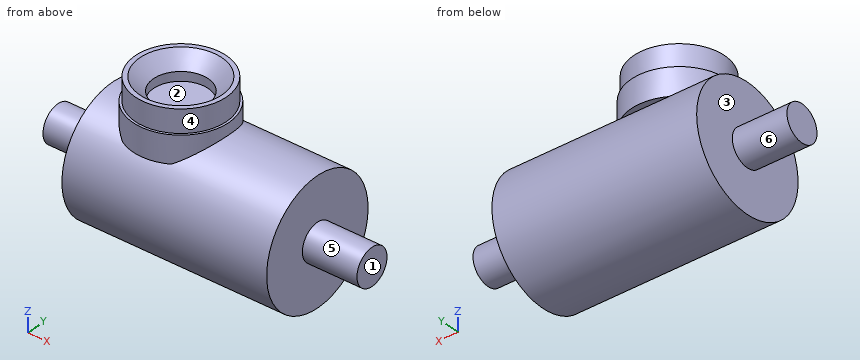
Autodesk Inventor part; units mm, degrees
ref_plane "Płaszczyzna konstrukcyjna1" through (0, 0, 10) normal (0, 0, 1) x (1, 0, 0)
ref_plane "YZ Plane" through (0, 0, 0) normal (1, 0, 0) x (0, 1, 0)
ref_plane "XZ Plane" through (0, 0, 0) normal (0, 1, 0) x (-1, 0, 0)
sketch "Szkic1" plane through (0, 0, 0) normal (1, 0, 0) x (0, 1, 0)
  circle A0 centre (0, 0) radius 13.5
  dimension "d0" = 27
extrude "Wyciągnięcie proste1" add sketch "Szkic1" along normal mid plane 45
sketch "Szkic2" plane through (22.5, 0, 0) normal (1, 0, 0) x (0, 0, -1)
  circle A0 centre (0, 0) radius 4
  dimension "d3" = 8
extrude "Wyciągnięcie proste2" add sketch "Szkic2" along normal blind 12
mirror "Odbij1" about plane through (0, 0, 0) normal (1, 0, 0) of "Wyciągnięcie proste2"
ref_plane "Płaszczyzna konstrukcyjna1" through (0, 0, 10) normal (0, 0, 1) x (1, 0, 0)
sketch "Szkic3" plane through (0, 0, 10) normal (0, 0, 1) x (1, 0, 0)
  circle A0 centre (-7.5, 0) radius 10.5
  line L0 (-22.5, 13.5) -> (-22.5, -13.5)
  point P0 (0, 0)
  dimension "d7" = 21
  dimension "d8" = 15
  dimension "d9" = 13.5
extrude "Wyciągnięcie proste3" add sketch "Szkic3" along normal blind 6
sketch "Szkic4" plane through (-7.5, 0, 16) normal (0, 0, 1) x (1, 0, 0)
  circle A0 centre (0, 0) radius 10
  line L0 (-15, 13.5) -> (-15, -13.5)
  circle A1 centre (0, 0) radius 6
  point P0 (7.5, 0)
  dimension "d12" = 20
  dimension "d13" = 15
  dimension "d14" = 13.5
  dimension "d15" = 12
extrude "Wyciągnięcie proste4" add sketch "Szkic4" along normal blind 5
chamfer "Faza1" distance 3 angle 45 1 edges at (-13.5, 0, 21)
properties part number "Kamera" material "Tworzywo sztuczne ABS"
Build history of the part. All positions in model axes, mm. Face numbers are marked on the shaded views. A direction names the side the tool comes from. Coordinates: 2 decimals unless noted, no trailing zeros. Order: outer loops, then holes, each group sorted by start corner. A loop starts at its lowest first (then second) coordinate and runs counter-clockwise, first axis right, second up. Notation, with made-up numbers: (18.25, -21) - (73.25, -21) arc R29 cw to (73.25, 1) - close; hole circle Ø10 at (25.5, 53.5). An arc over 180 degrees is marked (long way). Put each result on its own line as item: value.
1. Saw through at A-A (y = 0). Write the cut outline in (x, z).
Answer sheet:
outline: (-34.5, -4) - (-22.5, -4) - (-22.5, -13.5) - (22.5, -13.5) - (22.5, -4) - (34.5, -4) - (34.5, 4) - (22.5, 4) - (22.5, 13.5) - (3, 13.5) - (3, 16) - (2.5, 16) - (2.5, 21) - (1.5, 21) - (-1.5, 18) - (-1.5, 16) - (-13.5, 16) - (-13.5, 18) - (-16.5, 21) - (-17.5, 21) - (-17.5, 16) - (-18, 16) - (-18, 13.5) - (-22.5, 13.5) - (-22.5, 4) - (-34.5, 4) - close
2. Saw through at C-C (x = 12.5). Write the cut outline in (y, z).
Answer sheet:
outline: circle Ø27 at (0, 0)
3. Saw through at D-D (z = -5.5). Write the cut outline in (x, y).
Answer sheet:
outline: (-22.5, -12.33) - (22.5, -12.33) - (22.5, 12.33) - (-22.5, 12.33) - close
4. Saw through at B-B (z = 0). Write the cut outline in (x, y), and give its area (3 significant figures).
Answer sheet:
outline: (-34.5, -4) - (-22.5, -4) - (-22.5, -13.5) - (22.5, -13.5) - (22.5, -4) - (34.5, -4) - (34.5, 4) - (22.5, 4) - (22.5, 13.5) - (-22.5, 13.5) - (-22.5, 4) - (-34.5, 4) - close
area: 1,410 mm^2
5. Pull direction X, two halves, no side cores. Call the marked faces 1, 2 and 3: pulls with the +X half, pulls with the -X half, needs draft (parallel to the pull), parting line crosses it, or undercut.
Answer sheet:
face 1: pulls with the +X half
face 2: undercut
face 3: pulls with the -X half
6. Drop flat-ended pins along their axis: P1, Ø9.5, axis at x = -7.5, y = 0, coming from the +Z side; P2, Ø8, axis at y = 0.5, z = -5.5, coming from the +X side; P3, Ø8, axis at x = -20.5, z = 12.5, coming from the +Y side; P4, Ø1.1, axis at x = -9.5, y = 9.5, coming from the -Z side. Give the stop position or say it passes through.
Answer sheet:
P1: stops at z = 16
P2: stops at x = 34.5
P3: stops at y = 10.49
P4: stops at z = -10.11
7. Tool access for the marked faces 4, 5 and 6: list every direction of +Z, -Z, +X, -X, +Y, -Y with a clear straight run to the whole face (end or side of a thin tool).
Answer sheet:
face 4: +Z
face 5: +X
face 6: -X
8. Probe line 1 along Y through (x, z) = (-7.5, 17.55); line 2 along X through (y, z) = (9, 5); line 3 along Z through (x, y) = (31.5, -1.5). List the from-to ranges inside material, lowest first. Write a range as [from, to].
Answer sheet:
line 1: y = [-10, -6], [6, 10]
line 2: x = [-22.5, 22.5]
line 3: z = [-3.71, 3.71]
